Part model, mm, in its own coordinate system. Face numbers are marked on the shaded views. Give positions to 0.01 mm unless a question says otherwise; leave off trailing zeros. Order: outer loops, then holes, each group sorted by start corner. A loop starts at its lowest first (then second) coordinate and runs counter-clockwise, first axis right, second up. Notation, with made-up numbers: (-11, -34) - (19, -34) arc R15 ccw to (19, -12) - close; hole circle Ø5 at (-26.75, 20). An arc over 180 degrees is marked (long way). One line per item, written item: value.
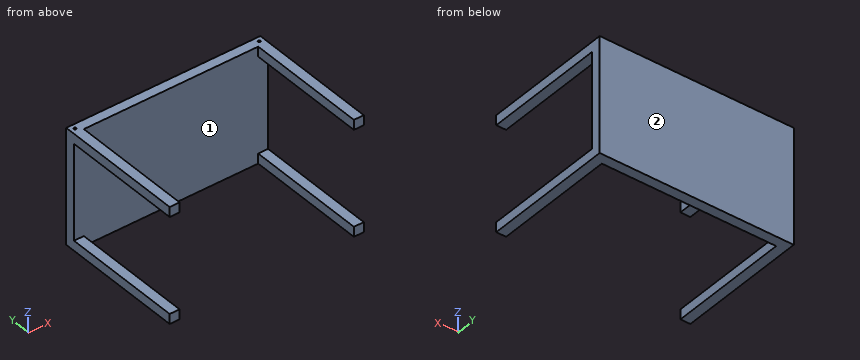
```python
from build123d import *

# Parameters (mm, degrees)
ESQUISSE1_W             = 1180
ESQUISSE1_H             = 800
BOSS_EXTRU_1_DEPTH      = 700
ESQUISSE2_W             = 1060
ESQUISSE2_H             = 740
ENL_V_MAT_EXTRU_1_DEPTH = 700
ESQUISSE3_W             = 580
ESQUISSE3_H             = 740
ENL_V_MAT_EXTRU_2_DEPTH = 1240
ESQUISSE7_R             = 7.5
ENL_V_MAT_EXTRU_5_DEPTH = 50


with BuildPart() as part:
    # Esquisse1 → Boss.-Extru.1 (new body)
    with BuildSketch(Plane.XY):
        with Locations((590, 400)):
            Rectangle(ESQUISSE1_W, ESQUISSE1_H)
    extrude(amount=BOSS_EXTRU_1_DEPTH)

    # Esquisse2 → Enlèv. mat.-Extru.1 (cut)
    with BuildSketch(Plane.XY.offset(700)):
        with Locations((590, 370)):
            Rectangle(ESQUISSE2_W, ESQUISSE2_H)
    extrude(amount=-ENL_V_MAT_EXTRU_1_DEPTH, mode=Mode.SUBTRACT)

    # Esquisse3 → Enlèv. mat.-Extru.2 (cut)
    with BuildSketch(Plane.ZY):
        with Locations((350, 370)):
            Rectangle(ESQUISSE3_W, ESQUISSE3_H)
    extrude(amount=-ENL_V_MAT_EXTRU_2_DEPTH, mode=Mode.SUBTRACT)

    # Esquisse7 → Enlèv. mat.-Extru.5 (cut)
    with BuildSketch(Plane.XY.offset(700)):
        with Locations((30, 770)):
            Circle(ESQUISSE7_R)
        with Locations((1150, 770)):
            Circle(ESQUISSE7_R)
    extrude(amount=-ENL_V_MAT_EXTRU_5_DEPTH, mode=Mode.SUBTRACT)


solid = part.part
```
1) Drill centre lines: line 1 along X through (y, z) = (770, 670); line 2 along Y through (x, z) = (1150, 668); line 3 along Y through (x, z) = (722, 623). Where is each one in solid material? Low to high. Write a range as from..to.
Outcome:
line 1: x = 0..22.5, 37.5..1142.5, 1157.5..1180
line 2: y = 0..762.5, 777.5..800
line 3: y = 740..800
2) Cut at B-B, the plane z = 588. Give the cut face in (x, y).
Outcome:
outline: (0, 740) - (1180, 740) - (1180, 800) - (0, 800) - close
3) Cut at A-A, the plane y = 219.5. Give the cut face in (x, z).
Outcome:
outline: (0, 0) - (60, 0) - (60, 60) - (0, 60) - close; (0, 640) - (60, 640) - (60, 700) - (0, 700) - close; (1120, 0) - (1180, 0) - (1180, 60) - (1120, 60) - close; (1120, 640) - (1180, 640) - (1180, 700) - (1120, 700) - close
4) Mould opens along X. For the marked faces 1 and 2 say: released by +X, released by -X, zero draft, split by the parting line, or undercut.
Outcome:
face 1: undercut
face 2: zero draft
5) Pin check, flat tips, straight feed: pin 1 (2 mm diameter, centred on x = 415.5, z = 167, fed in from -Y); pin 2 (9 mm diameter, centred on x = 1150, y = 770, fed in from +Z); pin 3 (18 mm diameter, centred on y = 407.5, z = 656, fed in from -X). Stop position of each tip, or through.
Outcome:
pin 1: stops at y = 740
pin 2: stops at z = 650
pin 3: stops at x = 0
6) Cut at C-C, the plane x = 615. Give the cut face in (y, z).
Outcome:
outline: (740, 0) - (800, 0) - (800, 700) - (740, 700) - close
